Verification items for the finished model (mm, model axes). Give positions to 0.01 mm unless a question says otherwise; leave off trailing zeros. Loops run counter-clockwise (first coordinate to the right, second up) from the corner with the lowest first, then second, coordinate; pieces in that order, holes last. Notation, with made-up numbers: M 23,23 L 60,23 A24 ccw 60,49 Z; hole C -3.5,-40 d7. An arc over 180 degrees is marked long. Write each question's results on one line, items separated by ' | '. Start each with the question number.
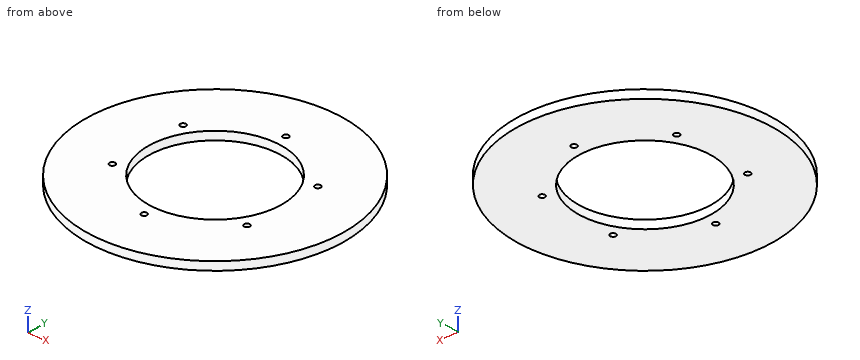
Solid Edge part; units mm, degrees
sketch "Sketch1" plane through (0, 0, 0) normal (0, 0, 1) x (1, 0, 0)
  circle A0 centre (0, 0) radius 111.23
  circle A1 centre (0, 0) radius 57.5
extrude "Protrusion1" add sketch "Sketch1" against normal blind 7.2
sketch "Sketch2" plane through (0, 0, 0) normal (0, 0, 1) x (1, 0, 0)
  circle A0 centre (0, 68) radius 2.46
extrude "Hål_för_skruv" cut sketch "Sketch2" along normal mid plane 644.3251
pattern_circular "Pattern1" count 6 over 360 about axis through (0, 0, 0) along (0, 0, -1) of "Hål_för_skruv"
properties material "Steel"
1. Section check B-B, the plane x = -16. Record the boundary of the cut face in (y, z).
2. Section check D-D, the plane y = -73. Record the boundary of the cut face in (x, z), plus the area to 3 significant figures.
3. Section check A-A, the plane y = 0. Record the boundary of the cut face in (x, z).
4. Thickness scan on probe 1 along Y at (x, z) = (0, -2.25); probe 2 along X at (y, z) = (32, -5.25); probe 3 along X at (y, z) = (-21.5, -5.5). Record the ranges inside material, lowest first.
5. Depth check by flat-ended pin: pin 1 Ø3 at (y, z) = (46.5, -5.5) entering from +X; pin 2 Ø4 at (y, z) = (82, -1) entering from +X; pin 3 Ø4 at (x, z) = (62, -5.5) entering from +Y. Enter the tip coordinate at first touch or a pass-through.
6. Section check C-C, the plane z = -3.5. Record the boundary of the cut face in (x, y).
Filled sheet:
1) outline: M -110.07,-7.2 L -55.23,-7.2 L -55.23,0 L -110.07,0 Z; M 55.23,-7.2 L 110.07,-7.2 L 110.07,0 L 55.23,0 Z
2) outline: M -83.92,-7.2 L 83.92,-7.2 L 83.92,0 L -83.92,0 Z | area: 1,210 mm2
3) outline: M -111.23,-7.2 L -57.5,-7.2 L -57.5,0 L -111.23,0 Z; M 57.5,-7.2 L 111.23,-7.2 L 111.23,0 L 57.5,0 Z
4) probe 1: -111.23 to -70.46, -65.54 to -57.5, 57.5 to 65.54, 70.46 to 111.23 | probe 2: -106.53 to -60.32, -57.46 to -47.77, 47.77 to 57.46, 60.32 to 106.53 | probe 3: -109.13 to -53.33, 53.33 to 109.13
5) pin 1: x = 101.72 | pin 2: x = 77.28 | pin 3: y = 93.66
6) outline: C 0,0 d222.46; hole C -58.89,-34 d4.92; hole C -58.89,34 d4.92; hole C 0,0 d115; hole C 0,-68 d4.92; hole C 0,68 d4.92; hole C 58.89,-34 d4.92; hole C 58.89,34 d4.92
